from build123d import *

# Parameters (mm, degrees)
SKETCH_R        = 47.5
PAD021_DEPTH    = 6
SKETCH017_R     = 2.2
POCKET013_DEPTH = 6.001
POCKET014_DEPTH = 2
FILLET_R        = 2.5
SKETCH024_R     = 10.5
POCKET036_DEPTH = 1


with BuildPart() as part:
    # Sketch → Pad021 (new body)
    with BuildSketch(Plane.XY):
        with BuildLine():
            Line((-59.336359, -41.65869), (-88.741901, -71.064232))
            Line((-88.741901, -71.064232), (-71.064232, -88.741901))
            Line((-71.064232, -88.741901), (-44.527821, -62.205491))
            ThreePointArc((-44.527821, -62.205491), (0, -76.5), (44.527821, -62.205491))
            Line((44.527821, -62.205491), (71.064232, -88.741901))
            Line((71.064232, -88.741901), (88.741901, -71.064232))
            Line((88.741901, -71.064232), (59.336359, -41.65869))
            ThreePointArc((59.336359, -41.65869), (72.5, 0), (59.336359, 41.65869))
            Line((100.838835, 83.161165), (59.336359, 41.65869))
            ThreePointArc((100.838835, 83.161165), (100.838835, 100.838835), (83.161165, 100.838835))
            Line((41.65869, 59.336359), (83.161165, 100.838835))
            ThreePointArc((41.65869, 59.336359), (0, 72.5), (-41.65869, 59.336359))
            Line((-83.161165, 100.838835), (-41.65869, 59.336359))
            ThreePointArc((-83.161165, 100.838835), (-100.838835, 100.838835), (-100.838835, 83.161165))
            Line((-59.336359, 41.65869), (-100.838835, 83.161165))
            ThreePointArc((-59.336359, 41.65869), (-72.5, 0), (-59.336359, -41.65869))
        make_face()
        Circle(SKETCH_R, mode=Mode.SUBTRACT)
        with BuildLine():
            ThreePointArc((-91.951086, 96.117962), (-96.862634, 94.777552), (-95.522224, 89.866004))
            Line((-95.522224, 89.866004), (-92.048914, 87.882038))
            ThreePointArc((-92.048914, 87.882038), (-87.137366, 89.222448), (-88.477776, 94.133996))
            Line((-91.951086, 96.117962), (-88.477776, 94.133996))
        make_face(mode=Mode.SUBTRACT)
        with BuildLine():
            ThreePointArc((95.522224, 89.866004), (96.862634, 94.777552), (91.951086, 96.117962))
            Line((91.951086, 96.117962), (88.477776, 94.133996))
            ThreePointArc((88.477776, 94.133996), (87.137366, 89.222448), (92.048914, 87.882038))
            Line((95.522224, 89.866004), (92.048914, 87.882038))
        make_face(mode=Mode.SUBTRACT)
        with BuildLine():
            ThreePointArc((-3.6, -66), (0, -69.6), (3.6, -66))
            Line((3.6, -66), (3.6, -62))
            ThreePointArc((3.6, -62), (0, -58.4), (-3.6, -62))
            Line((-3.6, -66), (-3.6, -62))
        make_face(mode=Mode.SUBTRACT)
    extrude(amount=PAD021_DEPTH)

    # Sketch017 (on DatumPlane) → Pocket013 (cut, through all)
    with BuildSketch(Plane.XY.offset(6)):
        with Locations((81.670833, -71.064232)):
            Circle(SKETCH017_R)
        with Locations((71.064232, -81.670833)):
            Circle(SKETCH017_R)
        with Locations((-71.064232, -81.670833)):
            Circle(SKETCH017_R)
        with Locations((-81.670833, -71.064232)):
            Circle(SKETCH017_R)
        with BuildLine():
            ThreePointArc((74.387633, 81.882965), (74.387633, 84.994235), (71.276364, 84.994235))
            Line((71.276364, 84.994235), (67.74083, 81.458701))
            ThreePointArc((67.74083, 81.458701), (67.74083, 78.347431), (70.852099, 78.347431))
            Line((74.387633, 81.882965), (70.852099, 78.347431))
        make_face()
        with BuildLine():
            ThreePointArc((84.994235, 71.276364), (84.994235, 74.387633), (81.882965, 74.387633))
            Line((81.882965, 74.387633), (78.347431, 70.852099))
            ThreePointArc((78.347431, 70.852099), (78.347431, 67.74083), (81.458701, 67.74083))
            Line((84.994235, 71.276364), (81.458701, 67.74083))
        make_face()
        with BuildLine():
            ThreePointArc((-71.276364, 84.994235), (-74.387633, 84.994235), (-74.387633, 81.882965))
            Line((-74.387633, 81.882965), (-70.852099, 78.347431))
            ThreePointArc((-70.852099, 78.347431), (-67.74083, 78.347431), (-67.74083, 81.458701))
            Line((-71.276364, 84.994235), (-67.74083, 81.458701))
        make_face()
        with BuildLine():
            ThreePointArc((-81.882965, 74.387633), (-84.994235, 74.387633), (-84.994235, 71.276364))
            Line((-84.994235, 71.276364), (-81.458701, 67.74083))
            ThreePointArc((-81.458701, 67.74083), (-78.347431, 67.74083), (-78.347431, 70.852099))
            Line((-81.882965, 74.387633), (-78.347431, 70.852099))
        make_face()
    extrude(amount=-POCKET013_DEPTH, mode=Mode.SUBTRACT)

    # Sketch012 (on DatumPlane) → Pocket014 (cut)
    with BuildSketch(Plane.XY.offset(6)):
        with BuildLine():
            ThreePointArc((6.5, -61.5), (0, -55), (-6.5, -61.5))
            Line((-6.5, -61.5), (-6.5, -66.5))
            ThreePointArc((-6.5, -66.5), (0, -73), (6.5, -66.5))
            Line((6.5, -61.5), (6.5, -66.5))
        make_face()
    extrude(amount=-POCKET014_DEPTH, mode=Mode.SUBTRACT)

    # Fillet
    fillet_edges = [part.edges().sort_by_distance(p)[0] for p in [
        (-59.336359, 41.65869, 3),
        (-59.336359, -41.65869, 3),
        (-88.741901, -71.064232, 3),
        (-84.994235, 71.276364, 3),
        (-74.387633, 81.882965, 3),
        (-71.276364, 84.994235, 3),
        (-81.882965, 74.387633, 3),
        (-44.527821, -62.205491, 3),
        (44.527821, -62.205491, 3),
        (59.336359, -41.65869, 3),
        (59.336359, 41.65869, 3),
        (41.65869, 59.336359, 3),
        (-41.65869, 59.336359, 3),
        (-71.064232, -88.741901, 3),
        (71.064232, -88.741901, 3),
        (88.741901, -71.064232, 3),
    ]]
    fillet(fillet_edges, radius=FILLET_R)

    # Sketch024 (on DatumPlane) → Pocket036 (cut)
    with BuildSketch(Plane.XY.offset(6)):
        with Locations((0, 60)):
            Circle(SKETCH024_R)
        with Locations((-51.961524, -30)):
            Circle(SKETCH024_R)
        with Locations((51.961524, -30)):
            Circle(SKETCH024_R)
    extrude(amount=-POCKET036_DEPTH, mode=Mode.SUBTRACT)


with BuildPart() as part_1:
    # Body placement: moved
    add(part.part.moved(Location((0, 0, -37))))


solid = part_1.part
Geometry: final body of the model. Coordinates: model frame, mm. A direction names the side the tool comes from. Give positions to 0.01 mm unless a question says otherwise; leave off trailing zeros. Write each loop counter-clockwise with the first axis right and the second up, starting at its lowest first coordinate (ties: lowest second). Pieces come first, ordered by that corner, then holes.
(1) Cut plane B-B, the plane x = 0. Return loops of the section in (y, z).
(2) Cut plane D-D, the plane y = -30. Return loops of the section in (x, z), then the cut area to 3 significant figures.
(3) Cut plane A-A, the plane y = 0. Return loops of the section in (x, z), then the cut area to 3 significant figures.
(4) Access query for faces 1 (the flat face through (-63.42, 81.1, -34.04)), 2 (the flat face through (-57.81, -75.49, -34.04)), 3 (the flat face through (-80.54, 62.86, -34.04)), 4 (the flat face through (-4, -64, -33)). Directions: +Z, -Z, +X, -X, +Y, -Y. A direction counts if a zero-diameter tool reaches every point of the face in a straight line with its end or side. Return the directions, or none.
(5) First-contact query: P1, Ø1.6, axis at y = -63.5, z = -32.5, coming from the -X side; P2, Ø5, axis at x = -81.67, y = -71.06, coming from the +Z side; P3, Ø0.6, axis at y = -63, z = -32, coming from the +X side. Flat tips, straight axial feed; report the tip coordinate or a pass-through.
(6) Ray query, line 1 (Y direction, x = 0.5, z = -36.1); line 2 (Y direction, x = -67, z = -31.5); line 3 (X direction, y = -26, z = -31.55). Return the intervals inside material, ascending.
(7) Mould query, pull axis X, two halves, no side actions, for faces 5 (the flat face through (-73.704, -56.026, -34.042)), 6 (the cylindrical face through (-1.37, 70.41, -31.49)), 7 (the cylindrical face through (72.498, -0.593, -34.042)), 8 (the cylindrical face through (87.1, 89.29, -34.04)). Classes: released by +X, released by -X, zero draft, split by the parting line, or undercut.
(8) Cut plane C-C, the plane x = -33.5. Return loops of the section in (y, z) (3 decimals), then the cut area to 3 significant figures.
Values follow:
1. outline: (-76.5, -37) - (-69.6, -37) - (-69.6, -33) - (-73, -33) - (-73, -31) - (-76.5, -31) - close; (-58.4, -37) - (-47.5, -37) - (-47.5, -31) - (-55, -31) - (-55, -33) - (-58.4, -33) - close; (47.5, -37) - (72.5, -37) - (72.5, -31) - (70.5, -31) - (70.5, -32) - (49.5, -32) - (49.5, -31) - (47.5, -31) - close
2. outline: (-66, -37) - (-36.83, -37) - (-36.83, -31) - (-41.46, -31) - (-41.46, -32) - (-62.46, -32) - (-62.46, -31) - (-66, -31) - close; (36.83, -37) - (66, -37) - (66, -31) - (62.46, -31) - (62.46, -32) - (41.46, -32) - (41.46, -31) - (36.83, -31) - close
2. area: 308 mm2
3. outline: (-72.5, -37) - (-47.5, -37) - (-47.5, -31) - (-72.5, -31) - close; (47.5, -37) - (72.5, -37) - (72.5, -31) - (47.5, -31) - close
3. area: 300 mm2
4. face 1: +Z, -Z, +Y
4. face 2: +Z, -Z, -Y
4. face 3: +Z, -Z, -X
4. face 4: +Z
5. P1: stops at x = -81.98
5. P2: stops at z = -31
5. P3: stops at x = 80.98
6. line 1: y = -76.5 to -69.57, -58.43 to -47.5, 47.5 to 72.5
6. line 2: y = -84.68 to -49.32, -27.7 to 27.7, 49.32 to 84.68
6. line 3: x = -67.68 to -61.67, -42.25 to -39.75, 39.75 to 42.25, 61.67 to 67.68
7. face 5: released by -X
7. face 6: undercut
7. face 7: released by +X
7. face 8: undercut
8. outline: (-68.775, -37) - (-33.675, -37) - (-33.675, -31) - (-68.775, -31) - close; (33.675, -37) - (64.296, -37) - (64.296, -31) - (33.675, -31) - close
8. area: 394 mm2
